Can you work these out from the model? Positions are in its coordinate system, mm. Face numbers are marked on the shaded views. A direction names the side the tool comes from. Coordinates: 2 decimals unless noted, no trailing zeros. Loops run counter-clockwise (first coordinate to the right, second up) from the corner with the lowest first, then second, coordinate; pieces in that order, holes last.
```python
from build123d import *

# Parameters (mm, degrees)
SKETCH1_W           = 12
SKETCH1_H           = 12
BOSS_EXTRUDE1_DEPTH = 37
SKETCH2_W           = 8
SKETCH2_H           = 8
CUT_EXTRUDE1_DEPTH  = 30
CUT_EXTRUDE2_REACH  = 39.961
SKETCH3_R           = 2.5


with BuildPart() as part:
    # Sketch1 → Boss-Extrude1 (new body)
    with BuildSketch(Plane.XY):
        Rectangle(SKETCH1_W, SKETCH1_H)
    extrude(amount=BOSS_EXTRUDE1_DEPTH)

    # Sketch2 → Cut-Extrude1 (cut)
    with BuildSketch(Plane(origin=(0, 0, 0), x_dir=(-1, 0, 0), z_dir=(0, 0, -1))):
        Rectangle(SKETCH2_W, SKETCH2_H)
    extrude(amount=-CUT_EXTRUDE1_DEPTH, mode=Mode.SUBTRACT)

    # Sketch3 → Cut-Extrude2 (cut, up to next)
    with BuildSketch(Plane.XY.offset(37), mode=Mode.PRIVATE) as cut_extrude2_sk1:
        Circle(SKETCH3_R)
    cut_extrude2_tool1 = extrude(cut_extrude2_sk1.sketch, amount=-CUT_EXTRUDE2_REACH, mode=Mode.PRIVATE) & part.part
    add(cut_extrude2_tool1.solids().sort_by_distance((0, 0, 37))[0], mode=Mode.SUBTRACT)


solid = part.part
```
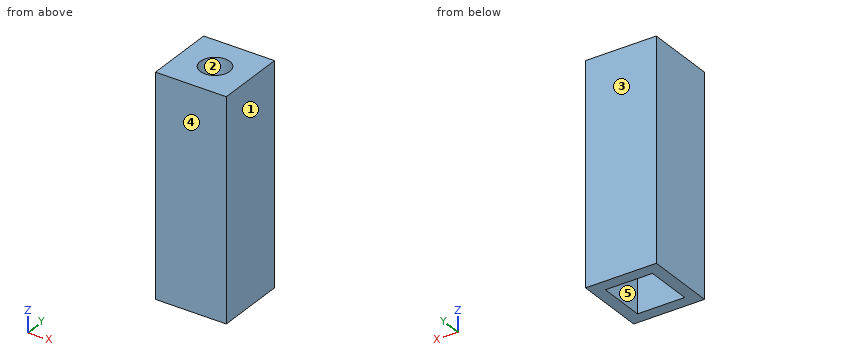
(1) I want a section at A-A on y = 0. Write out the boundary of the cut face in (x, z), then the cut area to 3 significant figures.
Check values:
outline: (-6, 0) - (-4, 0) - (-4, 30) - (-2.5, 30) - (-2.5, 37) - (-6, 37) - close; (2.5, 30) - (4, 30) - (4, 0) - (6, 0) - (6, 37) - (2.5, 37) - close
area: 169 mm2
(2) I want a section at D-D on x = 3. Write out the boundary of the cut face in (y, z).
Check values:
outline: (-6, 0) - (-4, 0) - (-4, 30) - (4, 30) - (4, 0) - (6, 0) - (6, 37) - (-6, 37) - close
(3) If we mould it in two halves opening along Y, with no side actions, what happens to the marked faces 1, 2 and 3? For each: released by +Y, released by -Y, zero draft, split by the parting line, or undercut.
Check values:
face 1: zero draft
face 2: undercut
face 3: released by +Y
(4) I'm going to push a flat-ended pin straight in: pin 1 (2.5 mm diameter, centred on x = 0.5, y = 1.5, fed in from -Z). Where does the tip first touch, or does it pass through?
Check values:
pin 1: stops at z = 30
(5) If I drill on probe 1 along X at (y, z) = (1, 21); probe 2 along Y at (x, z) = (0, 32.75), over which ranges is the centre line in solid material (lowest first)?
Check values:
probe 1: x = -6 to -4, 4 to 6
probe 2: y = -6 to -2.5, 2.5 to 6
(6) I want a section at B-B on z = 14. Write out the boundary of the cut face in (x, y), then the cut area to 3 significant figures.
Check values:
outline: (-6, -6) - (6, -6) - (6, 6) - (-6, 6) - close; hole (-4, -4) - (4, -4) - (4, 4) - (-4, 4) - close
area: 80.0 mm2
(7) Which directions (+Z, -Z, +X, -X, +Y, -Y) give clear straight access to the entire face, cutting with the end or side of a thin tool? Please do the marked faces 4 and 5.
Check values:
face 4: +Z, -Z, +X, -X, -Y
face 5: -Z
